```python
from build123d import *

# Parameters (mm, degrees)
SKETCH1_R           = 11.1125
SKETCH1_R_2         = 14.2875
SKETCH1_R_3         = 1.903475963
SKETCH1_R_4         = 2.0193
BOSS_EXTRUDE1_DEPTH = 6.35
FILLET1_R           = 25.4


with BuildPart() as part:
    # Sketch1 → Boss-Extrude1 (new body)
    with BuildSketch(Plane(origin=(0, 0, 0), x_dir=(0, 0, -1), z_dir=(1, 0, 0))):
        Polygon((0, 0), (0, 50.8), (228.6, 50.8), (255.540768363, 77.740768363), (306.340768363, 77.740768363), (333.281536726, 50.8), (381, 50.8), (381, 0), align=None)
        with Locations((25.4, 25.4)):
            Circle(SKETCH1_R, mode=Mode.SUBTRACT)
        with Locations((280.957536726, 52.340768363)):
            Circle(SKETCH1_R_2, mode=Mode.SUBTRACT)
        with Locations((355.6, 25.4)):
            Circle(SKETCH1_R_2, mode=Mode.SUBTRACT)
        with Locations((177.8, 25.4)):
            Circle(SKETCH1_R_2, mode=Mode.SUBTRACT)
        with Locations((304.762985996, 43.955677033)):
            Circle(SKETCH1_R_3, mode=Mode.SUBTRACT)
        with Locations((256.876798248, 60.913065482)):
            Circle(SKETCH1_R_4, mode=Mode.SUBTRACT)
    extrude(amount=BOSS_EXTRUDE1_DEPTH)

    # Fillet1
    fillet1_edges = [part.edges().sort_by_distance(p)[0] for p in [
        (3.175, 50.8, -228.6),
        (3.175, 50.8, -333.281536726),
        (3.175, 77.740768363, -306.340768363),
        (3.175, 77.740768363, -255.540768363),
        (3.175, 0, -381),
        (3.175, 50.8, -381),
        (3.175, 0, 0),
        (3.175, 50.8, 0),
    ]]
    fillet(fillet1_edges, radius=FILLET1_R - 0.0001)  # a hair under: the kernel refuses the full size


solid = part.part
```
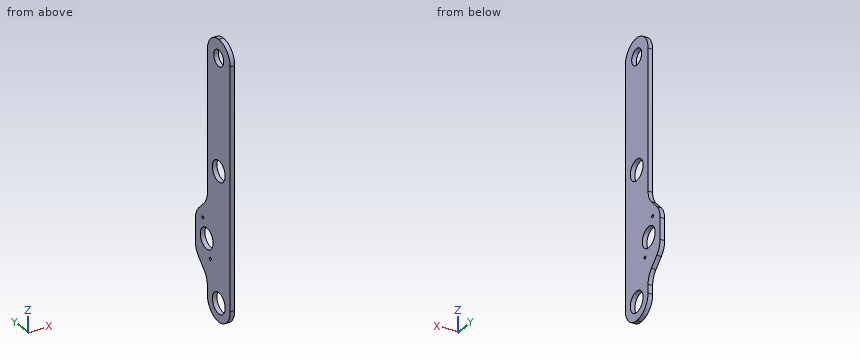
Input: part model. Units: mm. Frame: model coordinates. Give positions to 0.01 mm unless a question says otherwise; leave off trailing zeros. Order: outer loops, then holes, each group sorted by start corner. A loop starts at its lowest first (then second) coordinate and runs counter-clockwise, first axis right, second up. Notation, with made-up numbers: (26.5, -12.5) - (44.5, -12.5) arc R23 ccw to (44.5, 22.5) - close; hole circle Ø3 at (-19.5, 44.25). An arc over 180 degrees is marked (long way). One line per item, written item: value.
1. Pin query (flat end, axial travel): pin 1 Ø1 at (x, y) = (4.5, 31) entering from -Z; pin 2 Ø1.5 at (x, z) = (0.5, -140.5) entering from +Y; pin 3 Ø2 at (x, y) = (4, 54.5) entering from +Z. Return the tip coordinate at first contact, or that it passes through.
Determined:
pin 1: z = -380.48
pin 2: y = 50.8
pin 3: z = -229.48
2. Cut plane C-C, the plane x = 1.5. Give the number of separate pieces and of enclosed holes in the cut face, and give its area (3 significant figures).
Determined:
separate pieces: 1
enclosed holes: 6
area: 18,600 mm2
3. Cut plane D-D, the plane z = -78. Output: boundary loops of the cut face in (x, y).
Determined:
outline: (0, 0) - (6.35, 0) - (6.35, 50.8) - (0, 50.8) - close
4. Line query: probe 1 along Z at (x, y) = (2.75, 24.5); probe 2 along Z at (x, y) = (1, 18.5); probe 3 along Z at (x, y) = (6, 61). Output: solid intervals per line, ascending.
Determined:
probe 1: -380.98 to -369.86, -341.34 to -192.06, -163.54 to -36.48, -14.32 to -0.02
probe 2: -380.04 to -368.11, -343.09 to -190.31, -165.29 to -34.11, -16.69 to -0.96
probe 3: -323.08 to -292.32, -269.59 to -258.89, -254.86 to -238.8
5. Cut plane A-A, the plane z = -177.8. Output: boundary loops of the cut face in (x, y).
Determined:
outline: (0, 0) - (6.35, 0) - (6.35, 11.11) - (0, 11.11) - close; (0, 39.69) - (6.35, 39.69) - (6.35, 50.8) - (0, 50.8) - close
6. Cut plane B-B, the plane y = 32.5. Output: boundary loops of the cut face in (x, z).
Determined:
outline: (0, -379.99) - (6.35, -379.99) - (6.35, -368) - (0, -368) - close; (0, -343.2) - (6.35, -343.2) - (6.35, -190.2) - (0, -190.2) - close; (0, -165.4) - (6.35, -165.4) - (6.35, -33.95) - (0, -33.95) - close; (0, -16.85) - (6.35, -16.85) - (6.35, -1.01) - (0, -1.01) - close
